Build history of the part. All positions in model axes, mm. Give positions to 0.01 mm unless a question says otherwise; leave off trailing zeros. Write each loop counter-clockwise with the first axis right and the second up, starting at its lowest first coordinate (ties: lowest second). Pieces come first, ordered by that corner, then holes. Notation, with made-up numbers: (38, 70) -> (46, 70) arc R27 cw to (46, 91) -> close; hole circle Ø2 at (17.25, 9.25). An arc over 180 degrees is marked (long way). One line per question, with ' | ' between items. Start each with the question number.
(1) Pin check, flat tip, straight feed: P1, Ø1.2, axis at x = 17.25, y = -6.1, coming from the -Z side. Stop position of the tip, or through.
(2) Band-saw the part on B-B, the plane y = 17.9. Give the cut face in (x, z), and give its area (3 significant figures).
(3) Band-saw the part on D-D, the plane y = 26.5. Give the cut face in (x, z).
(4) Band-saw the part on C-C, the plane z = 0.75. Give the cut face in (x, y).
(5) Drill centre lines: probe 1 along X at (y, z) = (18, 0.55); probe 2 along Y at (x, z) = (0.5, 2.6); probe 3 along X at (y, z) = (-11.5, 1.2). Where is each one in solid material? Low to high. Write a range as from..to.
(6) Band-saw the part on A-A, the plane x = 0. Give the cut face in (y, z).
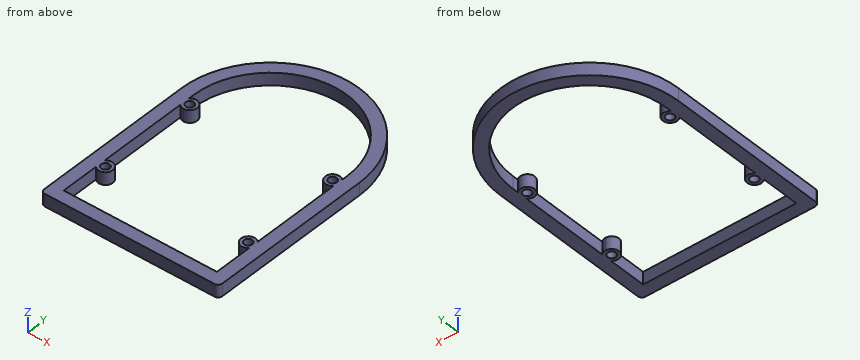
from build123d import *

# Parameters (mm, degrees)
SKETCH1_R           = 1
BOSS_EXTRUDE1_DEPTH = 3


with BuildPart() as part:
    # Sketch1 → Boss-Extrude1 (new body)
    with BuildSketch(Plane.XY):
        with BuildLine():
            ThreePointArc((21.5, 20.5), (0, 42), (-21.5, 20.5))
            Line((-21.5, 20.5), (-21.5, -18.5))
            ThreePointArc((-21.5, -18.5), (-21.207106781, -19.207106781), (-20.5, -19.5))
            Line((-20.5, -19.5), (20.5, -19.5))
            ThreePointArc((20.5, -19.5), (21.207106781, -19.207106781), (21.5, -18.5))
            Line((21.5, -18.5), (21.5, 20.5))
        make_face()
        with Locations((-17.25, -6.1)):
            Circle(SKETCH1_R, mode=Mode.SUBTRACT)
        with Locations((-17.25, 17.9)):
            Circle(SKETCH1_R, mode=Mode.SUBTRACT)
        with BuildLine():
            ThreePointArc((-18.5, -7.324744871), (-15.636648903, -6.77793675), (-17.25, -4.35))
            ThreePointArc((-17.25, -4.35), (-17.92793675, -4.486648903), (-18.5, -4.875255129))
            Line((-18.5, -4.875255129), (-18.5, 16.675255129))
            ThreePointArc((-18.5, 16.675255129), (-17.92793675, 16.286648903), (-17.25, 16.15))
            ThreePointArc((-17.25, 16.15), (-15.636648903, 18.57793675), (-18.5, 19.124744871))
            Line((-18.5, 19.124744871), (-18.5, 20.5))
            ThreePointArc((-18.5, 20.5), (0, 39), (18.5, 20.5))
            Line((18.5, 20.5), (18.5, 19.124744871))
            ThreePointArc((18.5, 19.124744871), (15.636648903, 18.57793675), (17.25, 16.15))
            ThreePointArc((17.25, 16.15), (17.92793675, 16.286648903), (18.5, 16.675255129))
            Line((18.5, 16.675255129), (18.5, -4.875255129))
            ThreePointArc((18.5, -4.875255129), (17.92793675, -4.486648903), (17.25, -4.35))
            ThreePointArc((17.25, -4.35), (15.636648903, -6.77793675), (18.5, -7.324744871))
            Line((18.5, -7.324744871), (18.5, -16.5))
            Line((18.5, -16.5), (-18.5, -16.5))
            Line((-18.5, -16.5), (-18.5, -7.324744871))
        make_face(mode=Mode.SUBTRACT)
        with Locations((17.25, 17.9)):
            Circle(SKETCH1_R, mode=Mode.SUBTRACT)
        with Locations((17.25, -6.1)):
            Circle(SKETCH1_R, mode=Mode.SUBTRACT)
    extrude(amount=BOSS_EXTRUDE1_DEPTH)


solid = part.part
Results:
1) P1: passes through
2) outline: (-21.5, 0) -> (-18.25, 0) -> (-18.25, 3) -> (-21.5, 3) -> close; (-16.25, 0) -> (-15.5, 0) -> (-15.5, 3) -> (-16.25, 3) -> close; (15.5, 0) -> (16.25, 0) -> (16.25, 3) -> (15.5, 3) -> close; (18.25, 0) -> (21.5, 0) -> (21.5, 3) -> (18.25, 3) -> close | area: 24.0 mm²
3) outline: (-20.65, 0) -> (-17.5, 0) -> (-17.5, 3) -> (-20.65, 3) -> close; (17.5, 0) -> (20.65, 0) -> (20.65, 3) -> (17.5, 3) -> close
4) outline: (-21.5, -18.5) arc R1 ccw to (-20.5, -19.5) -> (20.5, -19.5) arc R1 ccw to (21.5, -18.5) -> (21.5, 20.5) arc R21.5 ccw to (-21.5, 20.5) -> close; hole (-18.5, -16.5) -> (18.5, -16.5) -> (18.5, -7.32) arc R1.75 cw (long way) to (18.5, -4.88) -> (18.5, 16.68) arc R1.75 cw (long way) to (18.5, 19.12) -> (18.5, 20.5) arc R18.5 ccw to (-18.5, 20.5) -> (-18.5, 19.12) arc R1.75 cw (long way) to (-18.5, 16.68) -> (-18.5, -4.88) arc R1.75 cw (long way) to (-18.5, -7.32) -> close; hole circle Ø2 at (-17.25, -6.1); hole circle Ø2 at (-17.25, 17.9); hole circle Ø2 at (17.25, -6.1); hole circle Ø2 at (17.25, 17.9)
5) probe 1: x = -21.5..-18.24, -16.26..-15.5, 15.5..16.26, 18.24..21.5 | probe 2: y = -19.5..-16.5, 38.99..41.99 | probe 3: x = -21.5..-18.5, 18.5..21.5
6) outline: (-19.5, 0) -> (-16.5, 0) -> (-16.5, 3) -> (-19.5, 3) -> close; (39, 0) -> (42, 0) -> (42, 3) -> (39, 3) -> close
